```python
from build123d import *

# Parameters (mm, degrees)
SKETCH1_R           = 35
SKETCH1_R_2         = 23.425
SKETCH1_R_3         = 1.475
BOSS_EXTRUDE1_DEPTH = 2.5


with BuildPart() as part:
    # Sketch1 → Boss-Extrude1 (new, symmetric)
    with BuildSketch(Plane(origin=(0, 0, 0), x_dir=(1, 0, 0), z_dir=(0, 1, 0))):
        with Locations(Location((0, 0, 0), (0, 0, 270))):
            Circle(SKETCH1_R)
        with Locations(Location((0, 0, 0), (0, 0, 270))):
            Circle(SKETCH1_R_2, mode=Mode.SUBTRACT)
        with Locations(Location((-20.505, 20.505, 0), (0, 0, 270))):
            Circle(SKETCH1_R_3, mode=Mode.SUBTRACT)
        with Locations(Location((20.505, 20.505, 0), (0, 0, 90))):
            Circle(SKETCH1_R_3, mode=Mode.SUBTRACT)
        with Locations(Location((20.505, -20.505, 0), (0, 0, 270))):
            Circle(SKETCH1_R_3, mode=Mode.SUBTRACT)
        with Locations(Location((-20.505, -20.505, 0), (0, 0, 90))):
            Circle(SKETCH1_R_3, mode=Mode.SUBTRACT)
    extrude(amount=BOSS_EXTRUDE1_DEPTH, both=True)


solid = part.part
```
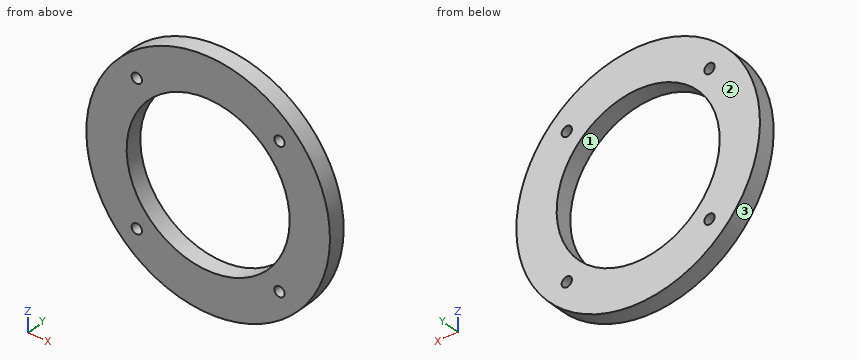
The model under review builds one solid part; all positions refer to its coordinate system, in mm. Face numbers are marked on the shaded views. Round coordinates to 2 decimals unless told otherwise and drop trailing zeros. Loops run counter-clockwise (first coordinate to the right, second up) from the corner with the lowest first, then second, coordinate; pieces in that order, holes last. Notation, with made-up numbers: (28.5, 51) - (37.5, 51) arc R17 ccw to (37.5, 60) - close; hole circle Ø8 at (-10.75, 75.25). An arc over 180 degrees is marked (long way). Use a Markdown table: item, result. Add a question column.
Q1. Insertion check: pin 1 Ø1 at (x, y) = (-21, 2) entering from +Z; pin 2 Ø1 at (x, y) = (-19, 0) entering from -Z; pin 3 Ø3 at (x, y) = (17, 0.5) entering from -Z. Each pin has a flat end and moves straight along its axis. Give the tip position at first contact, or say it passes through.
Q2. Add section D-D (y = 0.8). State the section outline as (x, z) points (3 decimals).
Q3. Add section B-B (x = 0). State the section outline as (y, z) points (3 decimals).
Q4. For probe 1 along X at (y, z) = (-0.15, 0) (3 decimals); probe 2 along Z at (x, y) = (3, -1.8); probe 3 along Z at (x, y) = (18, 0.75), list the stretches that pass through material, from the lowest coordinate up.
Q5. Add section A-A (z = 0). State the section outline as (x, y) points (3 decimals), plus the area to 3 significant figures.
Q6. Add section C-C (z = 21). State the section outline as (x, y) points, plus the area to 3 significant figures.
Q7. The part is to be moulded in two halves that separate along X. For the marked faces 1, 2 and 3, say which applies: pulls with the +X half, pulls with the -X half, needs draft (parallel to the pull), parting line crosses it, or undercut.
Worked answers:
| question | item | result |
|---|---|---|
| 1 | pin 1 | z = 28.37 |
| 1 | pin 2 | z = -29.71 |
| 1 | pin 3 | z = -31.38 |
| 2 | outline | circle Ø70 at (0, 0); hole circle Ø46.85 at (0, 0); hole circle Ø2.95 at (-20.505, -20.505); hole circle Ø2.95 at (-20.505, 20.505); hole circle Ø2.95 at (20.505, -20.505); hole circle Ø2.95 at (20.505, 20.505) |
| 3 | outline | (-2.5, -35) - (2.5, -35) - (2.5, -23.425) - (-2.5, -23.425) - close; (-2.5, 23.425) - (2.5, 23.425) - (2.5, 35) - (-2.5, 35) - close |
| 4 | probe 1 | -35 to -23.425, 23.425 to 35 |
| 4 | probe 2 | -34.87 to -23.23, 23.23 to 34.87 |
| 4 | probe 3 | -30.02 to -14.99, 14.99 to 30.02 |
| 5 | outline | (-35, -2.5) - (-23.425, -2.5) - (-23.425, 2.5) - (-35, 2.5) - close; (23.425, -2.5) - (35, -2.5) - (35, 2.5) - (23.425, 2.5) - close |
| 5 | area | 116 mm² |
| 6 | outline | (-28, -2.5) - (-21.89, -2.5) - (-21.89, 2.5) - (-28, 2.5) - close; (-19.12, -2.5) - (-10.38, -2.5) - (-10.38, 2.5) - (-19.12, 2.5) - close; (10.38, -2.5) - (19.12, -2.5) - (19.12, 2.5) - (10.38, 2.5) - close; (21.89, -2.5) - (28, -2.5) - (28, 2.5) - (21.89, 2.5) - close |
| 6 | area | 148 mm² |
| 7 | face 1 | undercut |
| 7 | face 2 | needs draft |
| 7 | face 3 | parting line crosses it |
